Design review of the part built by this model. Coordinates are the model's own, in mm. Face numbers are marked on the shaded views. A direction names the side the tool comes from. Round coordinates to 2 decimals unless told otherwise and drop trailing zeros. Write each loop counter-clockwise with the first axis right and the second up, starting at its lowest first coordinate (ties: lowest second). Pieces come first, ordered by that corner, then holes. Notation, with made-up numbers: (-38, -22) - (-30, -22) arc R31 cw to (-30, 14) - close; hole circle Ø7 at (22.5, 82). An arc over 180 degrees is marked (long way). Use one line per item in the form item = value.
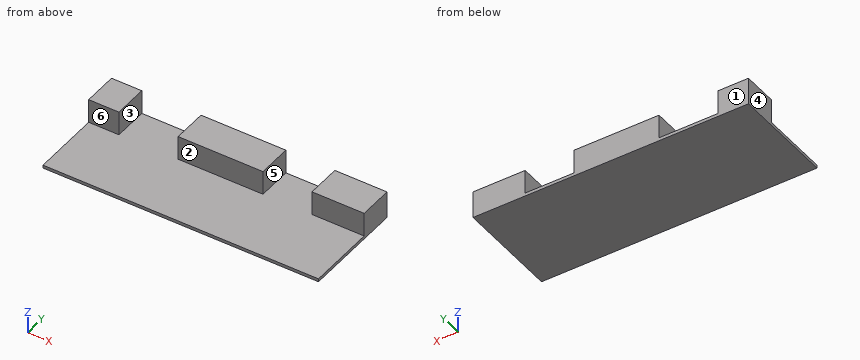
```python
from build123d import *

# Parameters (mm, degrees)
F0_W     = 1600
F0_H     = 600
F1_DEPTH = 18
F2_W     = 302.996802
F2_H     = 200
F2_W_2   = 492.690444
F2_W_3   = 175.781536
F3_DEPTH = 140


with BuildPart() as f1:
    # F0 (on Top) → F1 (new body)
    with BuildSketch(Plane.XY):
        Rectangle(F0_W, F0_H)
    extrude(amount=F1_DEPTH)

    # F2 (on face) → F3 (join)
    with BuildSketch(Plane.XY.offset(18)):
        with Locations((648.501599, 200)):
            Rectangle(F2_W, F2_H)
        with Locations((-33.959925, 200)):
            Rectangle(F2_W_2, F2_H)
        with Locations((-712.109232, 200)):
            Rectangle(F2_W_3, F2_H)
    extrude(amount=F3_DEPTH)


solid = f1.part
```
Q1. We need section C-C on x = -178. Write out the cut boundary in (y, z), then the cut area to 3 significant figures.
Calculated:
outline = (-300, 0) - (300, 0) - (300, 158) - (100, 158) - (100, 18) - (-300, 18) - close
area = 38,800 mm2
Q2. We need section A-A on z = 79. Write out the cut boundary in (x, y).
Calculated:
outline = (-800, 100) - (-624.22, 100) - (-624.22, 300) - (-800, 300) - close; (-280.31, 100) - (212.39, 100) - (212.39, 300) - (-280.31, 300) - close; (497, 100) - (800, 100) - (800, 300) - (497, 300) - close
Q3. To check wall thickness, follow line 1 along X through (y, z) = (103, 138); line 2 along Z through (x, y) = (169, 75.5); line 3 along Y through (x, z) = (633.5, 133.5). State the ranges of each line that lie inside material, in increasing order. Write a range as from..to.
Calculated:
line_1 = -800..-624.22, -280.31..212.39, 497..800
line_2 = 0..18
line_3 = 100..300
Q4. We need section D-D on x = 315.5. Write out the cut boundary in (y, z), then the cut area to 3 significant figures.
Calculated:
outline = (-300, 0) - (300, 0) - (300, 18) - (-300, 18) - close
area = 10,800 mm2
Q5. We need section B-B on y = 126. Write out the cut boundary in (x, z).
Calculated:
outline = (-800, 0) - (800, 0) - (800, 158) - (497, 158) - (497, 18) - (212.39, 18) - (212.39, 158) - (-280.31, 158) - (-280.31, 18) - (-624.22, 18) - (-624.22, 158) - (-800, 158) - close
Q6. Draft analysis for pull direction X (two halves, no side actions). For the marked faces 4, 5 and 6, state which applies: released by +X, released by -X, zero draft, split by the parting line, or undercut.
Calculated:
face_4 = released by -X
face_5 = undercut
face_6 = zero draft
Q7. For P1, Ø1, axis at x = 261, y = -189, coming from the +Z side; P2, Ø12, axis at x = 608, z = 70.5, coming from the -Y side, all flat-tipped, find the tip position at first contact; note any pin that passes through.
Calculated:
P1 = 18
P2 = 100
Q8. Machinability: for the marked faces 1, 2 and 3, which of the approach directions +Z, -Z, +X, -X, +Y, -Y give a long, thin tool a straight path to every point of the face, cutting with its end or side? Answer none if there is none.
Calculated:
face_1 = +Z, -Z, +X, -X, +Y
face_2 = +Z, +X, -X, -Y
face_3 = +Z, +Y, -Y
